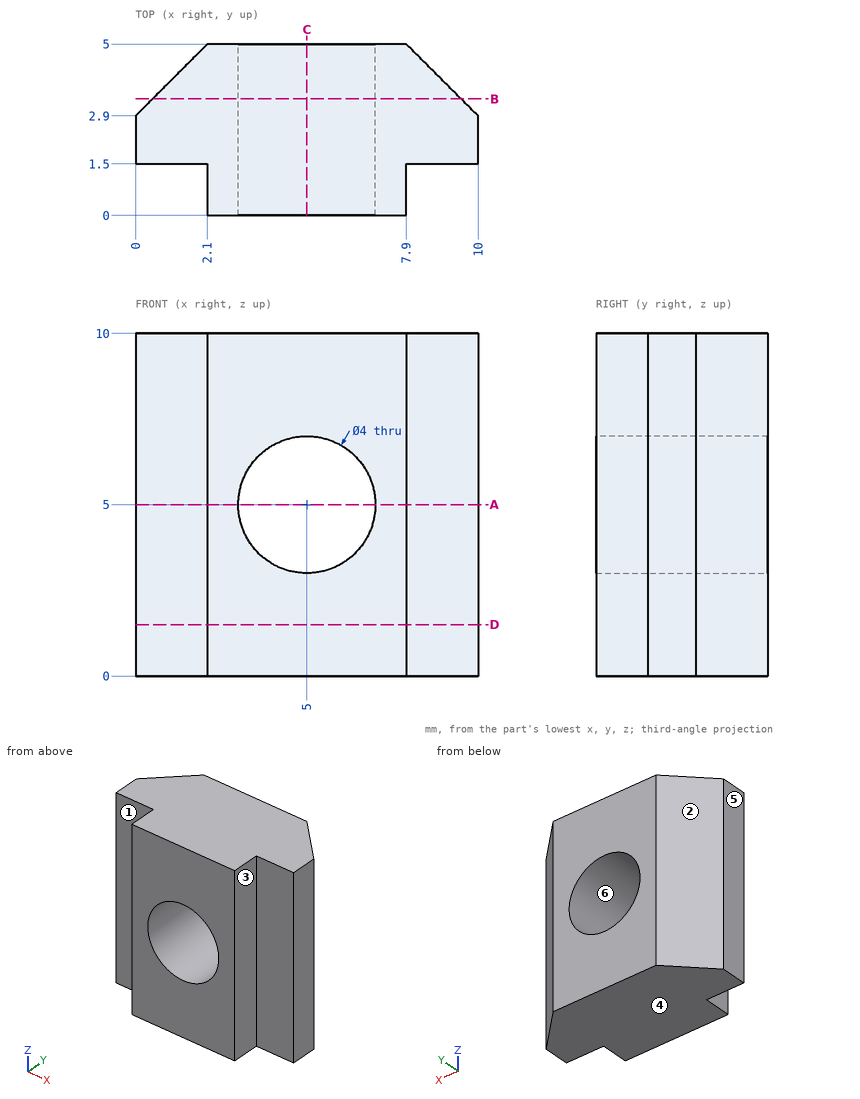
Design review of the part shown in the three views and the two pictorial views. Dimensions are in mm from the part's minimum x, y and z. A direction names the side the tool comes from. Give positions to 0.01 mm unless a question says otherwise; leave off trailing zeros. Write each loop counter-clockwise with the first axis right and the second up, starting at its lowest first coordinate (ties: lowest second). Pieces come first, ordered by that corner, then holes. Notation, with made-up numbers: M 42.25,-11.75 L 71.25,-11.75 A21 cw 71.25,-2.75 Z; hole C 35.5,2.5 d2. An arc over 180 degrees is marked long. Answer in a Markdown table with one row per item.
Item 1: For line 1 along X through (y, z) = (1.9, 5); line 2 along Z through (x, y) = (4.5, 4.4); line 3 along X through (y, z) = (1.25, 5), list the stretches that pass through material, from the lowest coordinate up.
Check sheet entries:
| item | result |
|---|---|
| line 1 | 0 to 3, 7 to 10 |
| line 2 | 0 to 3.06, 6.94 to 10 |
| line 3 | 2.1 to 3, 7 to 7.9 |
Item 2: Add section B-B on y = 3.4. Give the boundary of the cut face in (x, z).
Check sheet entries:
| item | result |
|---|---|
| outline | M 0.5,0 L 9.5,0 L 9.5,10 L 0.5,10 Z; hole C 5,5 d4 |
Item 3: Draft analysis for pull direction Z (two halves, no side actions). For the marked faces 4, 5 and 6, state which applies: +Z half, -Z half, draft (parallel to the pull), parting line (faces both ways), or undercut.
Check sheet entries:
| item | result |
|---|---|
| face 4 | -Z half |
| face 5 | draft |
| face 6 | undercut |
Item 4: Add section C-C on x = 5. Give the boundary of the cut face in (y, z), plus the area to 3 significant figures.
Check sheet entries:
| item | result |
|---|---|
| outline | M 0,0 L 5,0 L 5,3 L 0,3 Z; M 0,7 L 5,7 L 5,10 L 0,10 Z |
| area | 30.0 mm2 |
Item 5: For P1, Ø3, axis at y = 3.5, z = 1.5, coming from the -X side; P2, Ø0.8, axis at y = 1, z = 3.5, coming from the +X side; P3, Ø0.6, axis at x = 0.5, z = 7, coming from the -Y side; P4, Ø1.2, axis at y = 0.5, z = 5.5, coming from the -X side, all flat-tipped, find the tip position at first contact; note any pin that passes through.
Check sheet entries:
| item | result |
|---|---|
| P1 | x = 0 |
| P2 | x = 7.9 |
| P3 | y = 1.5 |
| P4 | x = 2.1 |
Item 6: Tool access review of the marked faces 1, 2 and 3: name each direction out of +Z, -Z, +X, -X, +Y, -Y from which nothing blocks a thin tool from reaching the whole face with its end or side.
Check sheet entries:
| item | result |
|---|---|
| face 1 | +Z, -Z, -X, -Y |
| face 2 | +Z, -Z, -X, +Y |
| face 3 | +Z, -Z, +X, -Y |
Item 7: Add section A-A on z = 5. Give the boundary of the cut face in (x, y).
Check sheet entries:
| item | result |
|---|---|
| outline | M 0,1.5 L 2.1,1.5 L 2.1,0 L 3,0 L 3,5 L 2.1,5 L 0,2.9 Z; M 7,0 L 7.9,0 L 7.9,1.5 L 10,1.5 L 10,2.9 L 7.9,5 L 7,5 Z |
Item 8: Add section D-D on z = 1.5. Give the boundary of the cut face in (x, y).
Check sheet entries:
| item | result |
|---|---|
| outline | M 0,1.5 L 2.1,1.5 L 2.1,0 L 7.9,0 L 7.9,1.5 L 10,1.5 L 10,2.9 L 7.9,5 L 2.1,5 L 0,2.9 Z |
